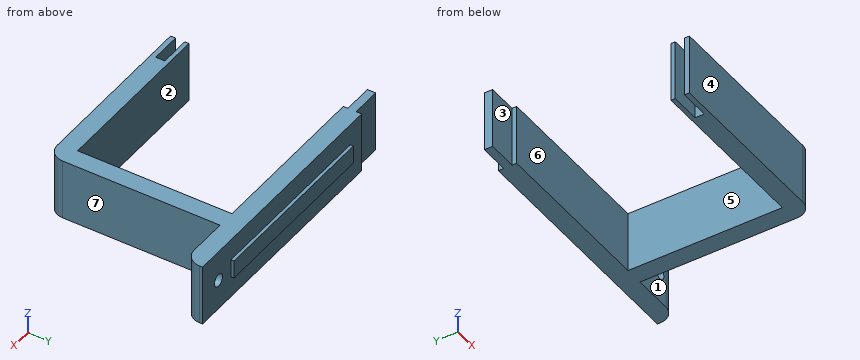
```python
from build123d import *

# Parameters (mm, degrees)
F0_W     = 112
F0_H     = 50.5
F1_DEPTH = 20
F2_R     = 5
F4_D     = 4.1
F6_DEPTH = 20
F7_W     = 60
F7_H     = 6
F8_DEPTH = 1


with BuildPart() as f1:
    # F0 (on Top) → F1 (new body)
    with BuildSketch(Plane.XY):
        Polygon((80, 3), (-80, 3), (-80, -3), (-62, -3), (-62, -59.5), (62, -59.5), (62, -3), (80, -3), align=None)
        with Locations((0, -28.25)):
            Rectangle(F0_W, F0_H, mode=Mode.SUBTRACT)
    extrude(amount=F1_DEPTH)

    # F2
    f2_edges = [f1.edges().sort_by_distance(p)[0] for p in [
        (62, -59.5, 10),
        (-62, -59.5, 10),
        (-80, -3, 10),
        (80, -3, 10),
    ]]
    fillet(f2_edges, radius=F2_R)

    # F4 (through all)
    with Locations(Plane(origin=(0, 3, 0), x_dir=(-1, 0, 0), z_dir=(0, 1, 0))):
        with Locations((-72, 10), (72, 10)):
            Hole(F4_D / 2)

    # F5 (on face) → F6 (cut, through all)
    with BuildSketch(Plane.XY.offset(20)):
        with BuildLine():
            Line((10, -57.87533), (10, -54.87533))
            Line((10, -54.87533), (0, -54.87533))
            Line((0, -54.87533), (0, -53.5))
            Line((0, -53.5), (-56, -53.5))
            Line((-56, -53.5), (-56, -3))
            Line((-56, -3), (0, -3))
            Line((0, -3), (0, -1.5))
            Line((0, -1.5), (-9.8, -1.5))
            Line((-9.8, -1.5), (-9.8, 1.2))
            Line((-9.8, 1.2), (0, 1.2))
            Line((0, 1.2), (0, 3))
            Line((0, 3), (-80, 3))
            Line((-80, 3), (-80, 2))
            ThreePointArc((-80, 2), (-78.535534, -1.535534), (-75, -3))
            Line((-75, -3), (-62, -3))
            Line((-62, -3), (-62, -54.5))
            ThreePointArc((-62, -54.5), (-60.535534, -58.035534), (-57, -59.5))
            Line((-57, -59.5), (0, -59.5))
            Line((0, -59.5), (0, -57.87533))
            Line((0, -57.87533), (10, -57.87533))
        make_face()
    extrude(amount=-F6_DEPTH, mode=Mode.SUBTRACT)

    # F7 (on face) → F8 (join)
    with BuildSketch(Plane(origin=(0, 3, 0), x_dir=(-1, 0, 0), z_dir=(0, 1, 0))):
        with Locations((-35.730945, 10)):
            Rectangle(F7_W, F7_H)
    extrude(amount=F8_DEPTH)


solid = f1.part
```
Design review of the part built by this model. Coordinates are the model's own, in mm. Face numbers are marked on the shaded views. A direction names the side the tool comes from. Round coordinates to 2 decimals unless told otherwise and drop trailing zeros. Write each loop counter-clockwise with the first axis right and the second up, starting at its lowest first coordinate (ties: lowest second). Pieces come first, ordered by that corner, then holes.
Item 1: For the marked faces 1, 2 and 3, list the 3-axis set-ups (+Z, -Z, +X, -X, +Y, -Y) from which the entire face can be reached by the end or side of a thin tool; tool diameter is ignored.
Item 2: For probe 1 along Y at (x, z) = (2, 9); probe 2 along Z at (x, y) = (72, 1); probe 3 along Y at (x, z) = (15, 11), list the stretches that pass through material, from the lowest coordinate up.
Item 3: Clearance check with flat-ended pins moving along their axes: pin 1 Ø4.5 at (x, z) = (72, 10) entering from -Y; pin 2 Ø8 at (y, z) = (-13, 15.5) entering from +X; pin 3 Ø1.1 at (y, z) = (3.5, 10) entering from -X. State where each tip first meets the part, or that it passes through.
Item 4: We need section B-B on z = 10. Write out the cut boundary in (x, y).
Item 5: We need section A-A on x = 72. Write out the cut boundary in (y, z), and give its area (3 significant figures).
Item 6: We need section D-D on x = -3. Write out the cut boundary in (y, z), and give its area (3 significant figures).
Item 7: The part is to be moulded in two halves that separate along Y. For the marked faces 4, 5, 6 and 7, say which applies: +Y half, -Y half, draft (parallel to the pull), parting line (faces both ways), or undercut.
Item 8: We need section C-C on z = 4.75. Write out the cut boundary in (x, y), and give its area (3 significant figures).
Returned:
1. face 1: +Z, -Z, +X, -Y
1. face 2: +Z, -Z, -X
1. face 3: +Z, -Z, -X, -Y
2. probe 1: y = -59.5 to -57.88, -54.88 to -53.5, -3 to 3
2. probe 2: z = 0 to 7.95, 12.05 to 20
2. probe 3: y = -59.5 to -53.5, -3 to 4
3. pin 1: stops at y = -3
3. pin 2: stops at x = 62
3. pin 3: stops at x = 0
4. outline: (-9.8, -1.5) - (0, -1.5) - (0, -3) - (56, -3) - (56, -53.5) - (0, -53.5) - (0, -54.88) - (10, -54.88) - (10, -57.88) - (0, -57.88) - (0, -59.5) - (57, -59.5) arc R5 ccw to (62, -54.5) - (62, -3) - (69.95, -3) - (69.95, 3) - (65.73, 3) - (65.73, 4) - (5.73, 4) - (5.73, 3) - (0, 3) - (0, 1.2) - (-9.8, 1.2) - close; (74.05, -3) - (75, -3) arc R5 ccw to (80, 2) - (80, 3) - (74.05, 3) - close
5. outline: (-3, 0) - (3, 0) - (3, 7.95) - (-3, 7.95) - close; (-3, 12.05) - (3, 12.05) - (3, 20) - (-3, 20) - close
5. area: 95.4 mm2
6. outline: (-1.5, 0) - (1.2, 0) - (1.2, 20) - (-1.5, 20) - close
6. area: 54.0 mm2
7. face 4: -Y half
7. face 5: undercut
7. face 6: undercut
7. face 7: draft
8. outline: (-9.8, -1.5) - (0, -1.5) - (0, -3) - (56, -3) - (56, -53.5) - (0, -53.5) - (0, -54.88) - (10, -54.88) - (10, -57.88) - (0, -57.88) - (0, -59.5) - (57, -59.5) arc R5 ccw to (62, -54.5) - (62, -3) - (75, -3) arc R5 ccw to (80, 2) - (80, 3) - (0, 3) - (0, 1.2) - (-9.8, 1.2) - close
8. area: 1,140 mm2
